Design review of the part built by this model. Coordinates are the model's own, in mm. Face numbers are marked on the shaded views. A direction names the side the tool comes from. Round coordinates to 2 decimals unless told otherwise and drop trailing zeros. Write each loop counter-clockwise with the first axis right and the second up, starting at its lowest first coordinate (ties: lowest second). Pieces come first, ordered by that corner, then holes. Notation, with made-up numbers: M -19,3 L 15,3 A16 cw 15,23 Z; hole C 2,-37.5 d8. An arc over 180 degrees is marked long. Use CSV: the item, a comma, the result in double quotes.
Autodesk Inventor part; units mm, degrees
ref_plane "YZ Plane" through (0, 0, 0) normal (1, 0, 0) x (0, 1, 0)
ref_plane "XZ Plane" through (0, 0, 0) normal (0, 1, 0) x (-1, 0, 0)
ref_plane "XY Plane" through (0, 0, 0) normal (0, 0, 1) x (1, 0, 0)
sketch "Sketch1" plane through (0, 0, 0) normal (0, 0, 1) x (1, 0, 0)
  line L0 (0, 0) -> (42, 0)
  line L1 (42, 0) -> (42, 26.724)
  line L2 (0, 26.724) -> (0, 26.724)
  line L3 (0, 26.724) -> (0, 0)
  line L4 (1, 26.724) -> (41, 26.724)
  line L5 (41, 27.724) -> (41, 32.724)
  line L6 (41, 32.724) -> (1, 32.724)
  line L7 (1, 32.724) -> (1, 27.724)
  line L8 (1, 27.724) -> (0, 26.724)
  line L9 (42, 26.724) -> (42, 26.724)
  line L10 (41, 27.724) -> (42, 26.724)
  point P0 (42, 26.724)
  dimension "d0" = 26.724
  dimension "d1" = 42
  dimension "d2" = 0
  dimension "d3" = 40
  dimension "d4" = 1
  dimension "d5" = 1
  dimension "d6" = 1
  dimension "d7" = 1
  dimension "d8" = 1
  dimension "d9" = 5
extrude "Extrusion1" add sketch "Sketch1" along normal blind 1.667
sketch "Sketch2" plane through (0, 0, 1.667) normal (0, 0, 1) x (1, 0, 0)
  line L0 (32.3, 4.2) -> (41, 4.2)
  line L1 (41, 4.2) -> (41, 0)
  line L2 (41, 0) -> (32.3, 0)
  line L3 (32.3, 0) -> (32.3, 4.2)
  line L4 (0, 0) -> (42, 0)
  line L5 (1, 32.724) -> (1, 27.724)
  line L6 (41, 27.724) -> (41, 32.724)
  dimension "d12" = 0
  dimension "d14" = 8.7
  dimension "d15" = 4.2
  dimension "d18" = 0
extrude "Extrusion2" cut sketch "Sketch2" against normal blind 2.083
sketch "Sketch3" plane through (0, 0, 1.667) normal (0, 0, 1) x (1, 0, 0)
  line L0 (41.75, 13.5) -> (39.75, 13.5)
  line L1 (39.75, 13.5) -> (39.75, 22.2)
  line L2 (39.75, 22.2) -> (41.75, 22.2)
  line L3 (41.75, 22.2) -> (41.75, 13.5)
  line L4 (0.25, 13.5) -> (2.25, 13.5)
  line L5 (2.25, 13.5) -> (2.25, 22.2)
  line L6 (2.25, 22.2) -> (0.25, 22.2)
  line L7 (0.25, 22.2) -> (0.25, 13.5)
  line L8 (0, 0) -> (32.3, 0)
  line L9 (0, 26.724) -> (0, 0)
  line L10 (42, 0) -> (42, 26.724)
  dimension "d19" = 13.5
  dimension "d20" = 0
  dimension "d21" = 22.2
  dimension "d22" = 0
  dimension "d23" = 0.25
  dimension "d24" = 0.25
  dimension "d25" = 2
  dimension "d26" = 2
extrude "Extrusion3" add sketch "Sketch3" along normal blind 3
sketch "Sketch4" plane through (0.25, 13.5, 1.667) normal (-1, 0, 0) x (0, 0, 1)
  line L0 (0, 8.7) -> (3, 8.7)
  line L1 (3, 8.7) -> (1.5, 8.7)
  line L2 (1.5, 8.7) -> (1.5, 0)
  line L3 (1.5, 0) -> (3, 0)
  line L4 (3, 0) -> (3, 8.7)
  line L5 (0, 0) -> (3, 0)
  line L6 (0, 13.224) -> (0, -13.5)
  point P0 (-1.667, -13.5)
  dimension "d29" = 0
  dimension "d30" = 1.5
extrude "Extrusion4" add sketch "Sketch4" along normal blind 1.25 contours L0 L4 L3 L2
sketch "Sketch5" plane through (41.75, 13.5, 1.667) normal (1, 0, 0) x (0, 0, -1)
  line L0 (-3, 0) -> (-3, 8.7)
  line L1 (-3, 8.7) -> (-1.5, 8.7)
  line L2 (-1.5, 8.7) -> (-1.5, 0)
  line L3 (-1.5, 0) -> (-3, 0)
  line L4 (-3, 0) -> (-3, 8.7)
  line L5 (0, -13.5) -> (0, 13.224)
  line L6 (0, 0) -> (-3, 0)
  point P0 (1.667, -13.5)
  dimension "d33" = 1.5
  dimension "d34" = 0
extrude "Extrusion5" add sketch "Sketch5" along normal blind 1.25
chamfer "Chamfer1" distance 1.25 angle 45 2 edges at (41.75, 17.85, 3.167) (0.25, 17.85, 3.167)
sketch "Sketch6" plane through (0, 0, 1.667) normal (0, 0, 1) x (1, 0, 0)
  line L0 (10.3, 4) -> (25.3, 4)
  line L1 (25.3, 4) -> (25.3, 9)
  line L2 (25.3, 9) -> (10.3, 9)
  line L3 (10.3, 9) -> (10.3, 4)
  line L4 (0, 0) -> (32.3, 0)
  line L5 (32.3, 0) -> (32.3, 4.2)
  dimension "d40" = 4
  dimension "d41" = 15
  dimension "d42" = 5
  dimension "d43" = 7
extrude "Extrusion6" add sketch "Sketch6" along normal blind 10
chamfer "Chamfer2" distance 1 angle 45 2 edges at (43, 17.85, 4.667) (-1, 17.85, 4.667)
fillet "Fillet1" radius 2 2 edges at (39.75, 17.85, 1.667) (2.25, 17.85, 1.667)
equation "\"d8\" = d7"
properties part number "eonPCBcover"
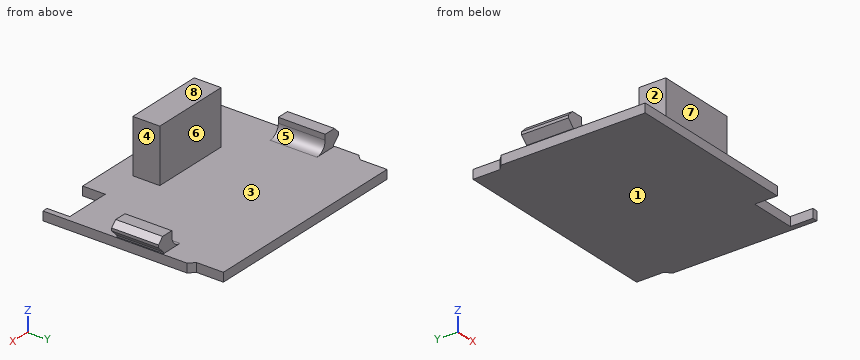
1) Add section A-A on x = 15.5. Write out the cut boundary in (y, z).
Answers:
outline,"M 0,0 L 32.72,0 L 32.72,1.67 L 9,1.67 L 9,11.67 L 4,11.67 L 4,1.67 L 0,1.67 Z"
2) Wall thickness on line 1 along Z through (x, y) = (21, 15.5); line 2 along X through (y, z) = (25, 1); line 3 along Y through (x, z) = (41.5, 3.25): over which ranges is each line inside the solid? List them lowest first. Write a range as [from, to].
Answers:
line 1,"[0, 1.67]"
line 2,"[0, 42]"
line 3,"[13.5, 22.2]"
3) The part is to be moulded in two halves that separate along X. For the marked faces 1, 2, 3 and 4, say which applies: released by +X, released by -X, zero draft, split by the parting line, or undercut.
Answers:
face 1,"zero draft"
face 2,"released by -X"
face 3,"undercut"
face 4,"released by +X"
4) For pin 1 Ø0.8 at (x, z) = (38.5, 0.5) entering from -Y; pin 2 Ø12 at (x, y) = (32.5, 18.5) entering from +Z; pin 3 Ø0.8 at (y, z) = (12.5, 1) entering from +X, all flat-tipped, find the tip position at first contact; note any pin that passes through.
Answers:
pin 1,"y = 4.2"
pin 2,"z = 1.81"
pin 3,"x = 42"
5) Machinability: for the marked faces 5, 6, 7 and 8, which of the approach directions +Z, -Z, +X, -X, +Y, -Y give a long, thin tool a straight path to every point of the face, cutting with its end or side? Answer none if there is none.
Answers:
face 5,"+Z, +Y, -Y"
face 6,"+Z, +X, -X, +Y"
face 7,"+Z, +X, -X, -Y"
face 8,"+Z, +X, -X, +Y, -Y"
6) Add section D-D on x = 9. Write out the cut boundary in (y, z).
Answers:
outline,"M 0,0 L 32.72,0 L 32.72,1.67 L 0,1.67 Z"
7) Add section C-C on z = 10. Write out the cut boundary in (x, y).
Answers:
outline,"M 10.3,4 L 25.3,4 L 25.3,9 L 10.3,9 Z"
8) Add section B-B on y = 5. Write out the cut boundary in (x, z).
Answers:
outline,"M 0,0 L 42,0 L 42,1.67 L 25.3,1.67 L 25.3,11.67 L 10.3,11.67 L 10.3,1.67 L 0,1.67 Z"
